Here's how the part is built. I have some questions about the finished solid (model axes, mm). A direction names the side the tool comes from. Coordinates: 2 decimals unless noted, no trailing zeros. Loops run counter-clockwise (first coordinate to the right, second up) from the corner with the lowest first, then second, coordinate; pieces in that order, holes last. Notation, with made-up numbers: (18.5, 58) -> (48.5, 58) arc R17 cw to (48.5, 91) -> close; hole circle Ø8 at (38, 1.5). An arc over 180 degrees is marked (long way). Answer as a JSON object with one key per item and string values. Group by question number.
1) I need wall thicknesses on probe 1 along Y at (x, z) = (-1.5, -1); probe 2 along X at (y, z) = (2.25, -2.25); probe 3 along X at (y, z) = (2, 2.75). Which ranges of each line are inside material? Lowest first, please. Write a range as [from, to].
2) I'm going to push flat-ended pins straight in: pin 1 (4 mm diameter, centred on y = 1, z = 1.5, fed in from +X); pin 2 (4 mm diameter, centred on x = 4, y = -1, fed in from -Z); pin 3 (3 mm diameter, centred on y = 2.5, z = 3, fed in from -X); pin 4 (0.7 mm diameter, centred on x = -1.5, z = 0, fed in from -Y). Where does each tip first touch, or does it pass through?
3) If we mould it in two halves opening along Z, with no side actions, what happens to faces 3 (the flat face through (8, 0, 0)), 4 (the cylindrical face through (-0.15, -2.8, -2.57)), 5 (the flat face through (-1.504, 0.616, -1.088))? For each: +Z half, -Z half, draft (parallel to the pull), parting line (faces both ways), or undercut.
4) Which directions (+Z, -Z, +X, -X, +Y, -Y) give clear straight access to the entire face, cutting with the end or side of a thin tool? Please do faces 1 (the cylindrical face through (4, 0, 2)), 2 (the flat face through (-2, 1.25, 0)).
5) I want a section at A-A (x = 6.25). Write out the boundary of the cut face in (y, z).
Autodesk Inventor part; units mm, degrees
ref_plane "Work Plane1" through (29, 0, 0) normal (0, -1, 0) x (1, 0, 0)
ref_plane "YZ Plane" through (0, 0, 0) normal (1, 0, 0) x (0, 1, 0)
ref_plane "XZ Plane" through (0, 0, 0) normal (0, 1, 0) x (-1, 0, 0)
sketch "Sketch1" plane through (0, 0, 0) normal (0, 0, 1) x (1, 0, 0)
  line L0 (-0.0667, 0) -> (8, 0)
  line L1 (8, 0) -> (8, 2)
  line L2 (8, 2) -> (1.4, 2)
  line L3 (1.4, 2) -> (0.9705, 2)
  line L4 (0.9705, 2) -> (0, 2)
  line L5 (0, 2) -> (0, 3.8)
  line L6 (0, 3.8) -> (-2.2, 3.8)
  line L7 (-2.2, 3.8) -> (-2.2, 1.4434)
  line L8 (-2.2, 1.4434) -> (-0.9, 1.4434)
  line L9 (-0.9, 1.4434) -> (-0.0667, 0)
  line L10 (-4.24, 0) -> (10.04, 0)
  line L11 (0, -0.76) -> (0, 4.56)
  line L12 (1.4, 2) -> (0, 2) construction
  dimension "d1" = 6.6
  dimension "d2" = 0.4295
  dimension "d3" = 2.2
  dimension "d4" = 1.3
  dimension "d5" = 60
  dimension "d6" = 4
  dimension "d7" = 4
  dimension "d8" = 2.8868
  dimension "d9" = 7.6
  dimension "d26" = 8
revolve "Body" add sketch "Sketch1" angle 360 about axis through (-0.0667, 0, 0) along (1, 0, 0)
sketch "Sketch2" plane through (-2.2, 0, 0) normal (-1, 0, 0) x (0, 0, 1)
  circle A0 centre (0, 0) radius 1.4434
  line L0 (0, -5.32) -> (0, 5.32)
  line L1 (-5.32, 0) -> (5.32, 0)
  line L2 (1.4434, 0) -> (0.7217, -1.25)
  line L3 (0.7217, -1.25) -> (-0.7217, -1.25)
  line L4 (-0.7217, -1.25) -> (-1.4434, 0)
  line L5 (-1.4434, 0) -> (-0.7217, 1.25)
  line L6 (-0.7217, 1.25) -> (0.7217, 1.25)
  line L7 (0.7217, 1.25) -> (1.4434, 0)
  point P0 (0, 0)
extrude "Slot" add sketch "Sketch2" against normal up to next contours L7 A0 | A0 L2 | L6 L0 A0 | A0 L0 L3 | L0 L6 A0 | A0 L3 L0 | L4 A0 | A0 L5
fillet "Fillet1" radius 1.9 1 edges at (-2.2, -3.8, 0)
thread "Thread"
chamfer "Chamfer1" distance 0.4294 distance2 0.4294 1 edges at (8, -2, 0) measured on face at (8, 0.556, 0.0273)
ref_plane "Work Plane1" through (29, 0, 0) normal (0, -1, 0) x (1, 0, 0)
fillet "Fillet2" radius 0.1 1 edges at (0, -2, 0)
equation "\"d1\" = GEL"
equation "\"d3\" = KOH"
equation "\"d4\" = INTI"
equation "\"d6\" = GD"
equation "\"d7\" = BDM"
equation "\"d8\" = 1.1547 * SW"
equation "\"d9\" = KOD"
equation "\"d26\" = NLG"
equation "\"d30\" = R"
equation "\"d17\" = RR"
equation "\"d13\" = GEL"
equation "\"d15\" = -0.5 * SPD + 0.5 * GD"
equation "\"d16\" = GUL"
equation "\"GD\" = NND"
equation "\"NLG\" = 8"
equation "\"GEL\" = 6.6"
equation "\"KOD\" = 7.6"
equation "\"KOH\" = 2.2"
equation "\"INTI\" = 1.3"
equation "\"GAL\" = 0.61345 * PTC"
equation "\"GUL\" = 0.61345 * PTC"
equation "\"BDM\" = NND"
equation "\"SW\" = 2.5"
equation "\"RR\" = 1.9"
equation "\"SPD\" = NND - 1.2269 * PTC"
equation "\"R\" = 0.1"
equation "\"TOA\" = 30deg"
equation "\"GD1\" = THREADDIA - 1.2269 * PTC"
equation "\"THREADDIA\" = 4"
equation "\"PTC\" = 0.7"
equation "\"NND\" = 4"
equation "\"KOH1\" = 0.3"
equation "\"E0\" = 1.155 * SW"
properties part number "BS 4168 - M4 x 8" material "Steel, Mild"
Determined:
{
 "1": {"probe 1": "[-3.22, -0.77], [0.77, 3.22]", "probe 2": "[-1.7, 0]", "probe 3": "[-1.47, 0]"},
 "2": {"pin 1": "x = 8", "pin 2": "z = -2", "pin 3": "x = -2.13", "pin 4": "y = -3.6"},
 "3": {"face 3": "draft", "face 4": "parting line", "face 5": "undercut"},
 "4": {"face 1": "+X", "face 2": "-X"},
 "5": {"outline": "circle Ø4 at (0, 0)"}
}
